Geometry check sheet. Reference: drawing and pictorial views, mm from the part's lowest x, y, z. A direction names the side the tool comes from. Round coordinates to 2 decimals unless told otherwise and drop trailing zeros. Order: outer loops, then holes, each group sorted by start corner. A loop starts at its lowest first (then second) coordinate and runs counter-clockwise, first axis right, second up.
Q1. Cross-section at C-C on x = 6.5. Record the cut outline in (y, z), then the cut area to 3 significant figures.
Q2. Scan lines: probe 1 along Z at (x, y) = (10, 4); probe 2 along Y at (x, z) = (16, 37.5); probe 3 along X at (y, z) = (7, 29.5). Record each from-to range of solid material in increasing order.
Q3. Cross-section at D-D on z = 25. Record the cut outline in (x, y).
Q4. Depth check by flat-ended pin: P1, Ø7.5, axis at x = 23.5, z = 15, coming from the +Y side; P2, Ø2, axis at y = 8, z = 24.5, coming from the -X side. Enter the tip coordinate at first touch or a pass-through.
Q5. Set-up check for the marked faces 1, 2 and 3: record each of +Z, -Z, +X, -X, +Y, -Y from which the full face is reachable in a straight line by a thin tool's end or side.
Q6. Cross-section at A-A on y = 9. Record the cut outline in (x, z).
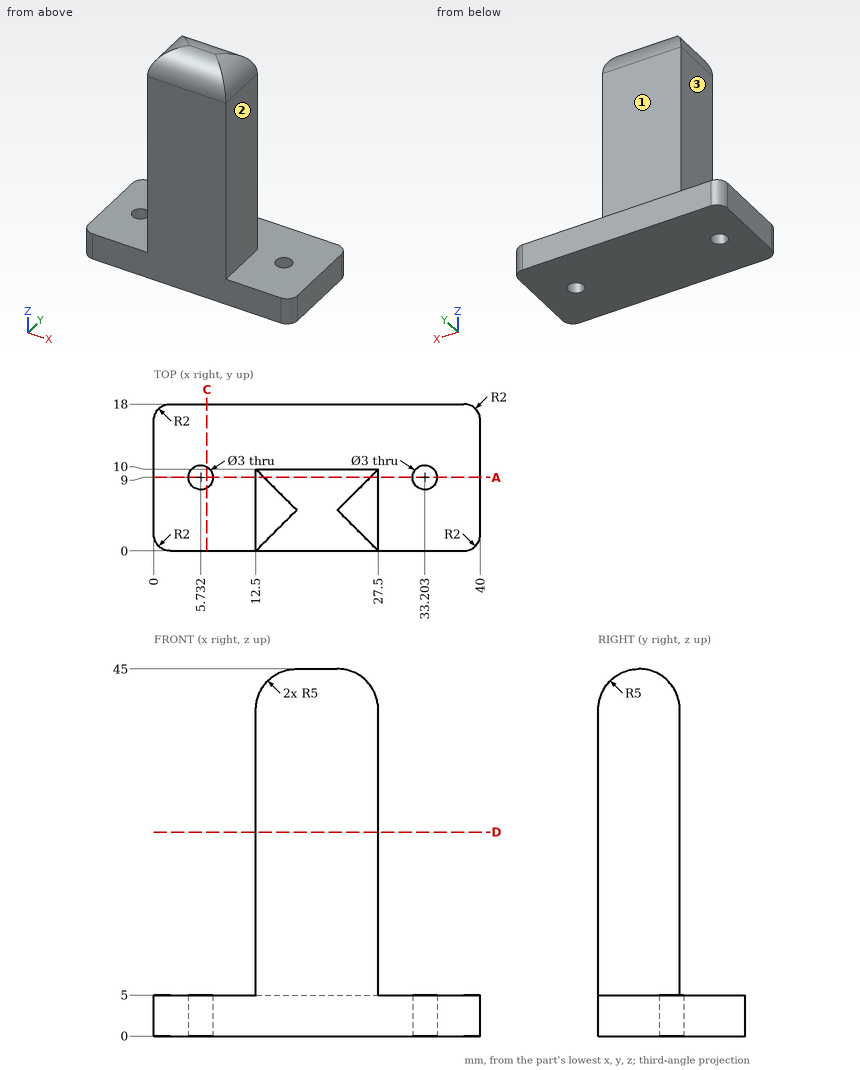
Results found:
1. outline: (0, 0) - (7.71, 0) - (7.71, 5) - (0, 5) - close; (10.29, 0) - (18, 0) - (18, 5) - (10.29, 5) - close
1. area: 77.1 mm2
2. probe 1: z = 0 to 5
2. probe 2: y = 0 to 10
2. probe 3: x = 12.5 to 27.5
3. outline: (12.5, 0) - (27.5, 0) - (27.5, 10) - (12.5, 10) - close
4. P1: stops at y = 10
4. P2: stops at x = 12.5
5. face 1: +Z, +X, -X, +Y
5. face 2: +Z, +X, +Y, -Y
5. face 3: +Z, -X, +Y, -Y
6. outline: (0, 0) - (4.23, 0) - (4.23, 5) - (0, 5) - close; (7.23, 0) - (31.7, 0) - (31.7, 5) - (27.5, 5) - (27.5, 40) arc R5 ccw to (26.5, 43) - (13.5, 43) arc R5 ccw to (12.5, 40) - (12.5, 5) - (7.23, 5) - close; (34.7, 0) - (40, 0) - (40, 5) - (34.7, 5) - close
